from build123d import *

# Parameters (mm, degrees)
SKETCH_W        = 70
SKETCH_H        = 50
PAD_DEPTH       = 5
SKETCH001_R     = 2.625
POCKET_DEPTH    = 5
SKETCH002_W     = 47
SKETCH002_H     = 50
PAD001_DEPTH    = 50
SKETCH003_W     = 36.5
SKETCH003_H     = 50
POCKET001_DEPTH = 50
POCKET002_DEPTH = 40
POCKET003_DEPTH = 50
SKETCH005_W     = 40
SKETCH005_H     = 5
PAD002_DEPTH    = 40
SKETCH006_R     = 2.625
POCKET004_DEPTH = 5
SKETCH007_W     = 30
SKETCH007_H     = 5
PAD003_DEPTH    = 10


with BuildPart() as part:
    # Sketch → Pad (new body)
    with BuildSketch(Plane.XY):
        Rectangle(SKETCH_W, SKETCH_H)
    extrude(amount=PAD_DEPTH)

    # Sketch001 (on Face6 of Pad) → Pocket (cut)
    with BuildSketch(Plane.XY.offset(5)):
        with Locations((-30, 20)):
            Circle(SKETCH001_R)
        with Locations((30, 20)):
            Circle(SKETCH001_R)
        with Locations((30, -20)):
            Circle(SKETCH001_R)
        with Locations((-30, -20)):
            Circle(SKETCH001_R)
    extrude(amount=-POCKET_DEPTH, mode=Mode.SUBTRACT)

    # Sketch002 (on Face5 of Pocket) → Pad001 (join)
    with BuildSketch(Plane.XY.offset(5)):
        Rectangle(SKETCH002_W, SKETCH002_H)
    extrude(amount=PAD001_DEPTH)

    # Sketch003 (on Face16 of Pad001) → Pocket001 (cut)
    with BuildSketch(Plane.XY.offset(55)):
        Rectangle(SKETCH003_W, SKETCH003_H)
    extrude(amount=-POCKET001_DEPTH, mode=Mode.SUBTRACT)

    # Sketch004 (on Face18 of Pocket001) → Pocket002 (cut)
    with BuildSketch(Plane.YZ.offset(23.5)):
        with BuildLine():
            Line((-8.332745, 55), (-1.252745, 47.92))
            ThreePointArc((-7.08, 42.08), (-1.246373, 42.086373), (-1.252745, 47.92))
            Line((-20, 55), (-7.08, 42.08))
            Line((-20, 55), (-8.332745, 55))
        make_face()
    extrude(amount=-POCKET002_DEPTH, mode=Mode.SUBTRACT)

    # Sketch004 (on Face18 of Pocket001) → Pocket003 (cut)
    with BuildSketch(Plane.YZ.offset(23.5)):
        with BuildLine():
            Line((-8.332745, 55), (-1.252745, 47.92))
            ThreePointArc((-7.08, 42.08), (-1.246373, 42.086373), (-1.252745, 47.92))
            Line((-20, 55), (-7.08, 42.08))
            Line((-20, 55), (-8.332745, 55))
        make_face()
    extrude(amount=-POCKET003_DEPTH, mode=Mode.SUBTRACT)

    # Sketch005 (on Face3 of Pocket003) → Pad002 (join)
    with BuildSketch(Plane(origin=(0, 25, 0), x_dir=(-1, 0, 0), z_dir=(0, 1, 0))):
        with Locations((-15, 2.5)):
            Rectangle(SKETCH005_W, SKETCH005_H)
    extrude(amount=PAD002_DEPTH)

    # Sketch006 (on Face21 of Pad002) → Pocket004 (cut)
    with BuildSketch(Plane.XY.offset(5)):
        with Locations((30, 60)):
            Circle(SKETCH006_R)
        with Locations((10, 60)):
            Circle(SKETCH006_R)
    extrude(amount=-POCKET004_DEPTH, mode=Mode.SUBTRACT)

    # Sketch007 (on Face3 of Pocket004) → Pad003 (join)
    with BuildSketch(Plane(origin=(0, 25, 0), x_dir=(-1, 0, 0), z_dir=(0, 1, 0))):
        with Locations((20, 2.5)):
            Rectangle(SKETCH007_W, SKETCH007_H)
    extrude(amount=PAD003_DEPTH)


solid = part.part
Geometry: final body of the model. Coordinates: model frame, mm. A direction names the side the tool comes from. Give positions to 0.01 mm unless a question says otherwise; leave off trailing zeros. Write each loop counter-clockwise with the first axis right and the second up, starting at its lowest first coordinate (ties: lowest second). Pieces come first, ordered by that corner, then holes. Notation, with made-up numbers: (-33, -17.5) - (-27, -17.5) arc R23 ccw to (-27, 12.5) - close; hole circle Ø3 at (17, -3.75). An arc over 180 degrees is marked (long way). Return JSON: item names as keys, results as strings. Group by question number.
1) Line query: line 1 (Y direction, x = -30, z = 1.5) (3 decimals); line 2 (Y direction, x = 30, z = 1) (3 decimals); line 3 (X direction, y = 6, z = 24.5). Output: solid intervals per line, ascending.
2) Section A-A on z = 45. Return the cut outline in (x, y), plus the area to 3 significant figures.
3) Mould query, pull axis X, two halves, no side actions, for faces 5 (the flat face through (20.91, -4.84, 51.51)), 6 (the flat face through (-5, 50, 2)), 7 (the cylindrical face through (28.065, -18.226, 2.535)). Classes: released by +X, released by -X, zero draft, split by the parting line, or undercut.
4) Set-up query: faces 1 (the flat face through (18.25, 0, 30)), 2 (the flat face through (-23.5, 0, 30)), 3 (the flat face through (21, 25, 30)), 4 (the flat face through (-20.84, -4.84, 51.51)). Return all of +Z, -Z, +X, -X, +Y, -Y with unobstructed straight access to the full face (end or side cutting, diameter ignored); none if empty.
5) Section C-C on y = 60. Return the cut outline in (x, z) (3 decimals), plus the area to 4 significant figures.
6) Section D-D on z = 32. Return the cut outline in (x, y), plus the area to 3 significant figures.
7) Section B-B on x = 10. Return the cut outline in (y, z) (3 decimals).
8) First-contact query: P1, Ø5, axis at x = 2, y = 53.5, coming from the +Z side; P2, Ø1.6, axis at x = 20.5, z = 18, coming from the +Y side; P3, Ø1.5, axis at y = 43, z = 2.5, coming from the -X side. Flat tips, straight axial feed; report the tip coordinate or a pass-through.
Filled in:
{
 "1": {"line 1": "y = -25 to -22.625, -17.375 to 17.375, 22.625 to 35", "line 2": "y = -25 to -22.625, -17.375 to 17.375, 22.625 to 57.375, 62.625 to 65", "line 3": "x = -23.5 to -18.25, 18.25 to 23.5"},
 "2": {"outline": "(-23.5, -25) - (-18.25, -25) - (-18.25, -10) - (-23.5, -10) - close; (-23.5, -0.04) - (-18.25, -0.04) - (-18.25, 25) - (-23.5, 25) - close; (18.25, -25) - (23.5, -25) - (23.5, -10) - (18.25, -10) - close; (18.25, -0.04) - (23.5, -0.04) - (23.5, 25) - (18.25, 25) - close", "area": "420 mm^2"},
 "3": {"face 5": "zero draft", "face 6": "released by -X", "face 7": "undercut"},
 "4": {"face 1": "+Z, +Y, -Y", "face 2": "+Z, -X, +Y, -Y", "face 3": "+Z, +X, -X, +Y", "face 4": "+X, -X"},
 "5": {"outline": "(-5, 0) - (7.375, 0) - (7.375, 5) - (-5, 5) - close; (12.625, 0) - (27.375, 0) - (27.375, 5) - (12.625, 5) - close; (32.625, 0) - (35, 0) - (35, 5) - (32.625, 5) - close", "area": "147.5 mm^2"},
 "6": {"outline": "(-23.5, -25) - (-18.25, -25) - (-18.25, 25) - (-23.5, 25) - close; (18.25, -25) - (23.5, -25) - (23.5, 25) - (18.25, 25) - close", "area": "525 mm^2"},
 "7": {"outline": "(-25, 0) - (57.375, 0) - (57.375, 5) - (-25, 5) - close; (62.625, 0) - (65, 0) - (65, 5) - (62.625, 5) - close"},
 "8": {"P1": "stops at z = 5", "P2": "stops at y = 25", "P3": "stops at x = -5"}
}
